Can you work these out from the model? Positions are in its coordinate system, mm. A direction names the side the tool comes from. Round coordinates to 2 decimals unless told otherwise and drop trailing zeros. Write each loop counter-clockwise with the first axis right and the second up, starting at its lowest first coordinate (ties: lowest second). Pieces come first, ordered by that corner, then holes. Notation, with made-up numbers: M 33.25,42 L 78.25,42 A13 cw 78.25,65 Z; hole C 42.5,12.25 d10. An arc over 180 degrees is marked long. Answer in a Markdown table with one row per item. Add a question column.
(1) I'm going to push flat-ended pins straight in: pin 1 (3 mm diameter, centred on y = -11, z = 32, fed in from +X); pin 2 (10 mm diameter, centred on x = 9.5, z = 8, fed in from +Y). Where does each tip first touch, or does it pass through?
(2) Suppose I cut it at C-C, the plane x = 12. Write out the boundary of the cut face in (y, z), then the cut area to 3 significant figures.
(3) If we mould it in two halves opening along Z, with no side actions, what happens to faces 3 (the face through (0, -7, 65)), 4 (the face through (32.5, -2, 32)), 5 (the face through (-2.48, -9, 33))? For each: released by +Z, released by -Z, zero draft, split by the parting line, or undercut.
(4) Suppose I cut it at D-D, the plane x = -16.5. Write out the boundary of the cut face in (y, z).
(5) If I drill on probe 1 along Z at (x, y) = (1, -7.75); probe 2 along Y at (x, z) = (24, 32.5); probe 3 along Y at (x, z) = (-1, 17.5), over which ranges is the centre line in solid material (lowest first)?
(6) For faces 1 (the face through (15.25, -7.44, 27.93)), 2 (the face through (0, -15, 32)), which set-ups out of +Z, -Z, +X, -X, +Y, -Y let a thin tool reach every point of the face, with its end or its side?
(7) Suppose I cut it at B-B, the plane z = 32.5. Write out the boundary of the cut face in (x, y), then the cut area to 3 significant figures.
(8) Suppose I cut it at A-A, the plane y = -8.88. Write out the boundary of the cut face in (x, z), then the cut area to 3 significant figures.
from build123d import *

# Parameters (mm, degrees)
SKIZZE1_W                       = 65
SKIZZE1_H                       = 30
AUFSATZ_LINEAR_AUSTRAGEN1_DEPTH = 65
SKIZZE2_R                       = 95
SCHNITT_LINEAR_AUSTRAGEN1_DEPTH = 65
SKIZZE5_R                       = 4.79
SCHNITT_LINEAR_AUSTRAGEN2_DEPTH = 34.98


with BuildPart() as part:
    # Skizze1 → Aufsatz-Linear austragen1 (new body)
    with BuildSketch(Plane.XY):
        Rectangle(SKIZZE1_W, SKIZZE1_H)
    extrude(amount=AUFSATZ_LINEAR_AUSTRAGEN1_DEPTH)

    # Skizze2 → Schnitt-Linear austragen1 (cut)
    with BuildSketch(Plane.XY.offset(65)):
        with Locations((0, 95)):
            Circle(SKIZZE2_R)
    extrude(amount=-SCHNITT_LINEAR_AUSTRAGEN1_DEPTH, mode=Mode.SUBTRACT)

    # Skizze5 → Schnitt-Linear austragen2 (cut)
    with BuildSketch(Plane(origin=(32.5, 0, 0), x_dir=(0, 0, -1), z_dir=(1, 0, 0))):
        with Locations((-32.5, -8.88)):
            Circle(SKIZZE5_R)
    extrude(amount=-SCHNITT_LINEAR_AUSTRAGEN2_DEPTH, mode=Mode.SUBTRACT)


solid = part.part
Calculated:
| question | item | result |
|---|---|---|
| 1 | pin 1 | x = -2.48 |
| 1 | pin 2 | y = 1.11 |
| 2 | outline | M -15,0 L 0.76,0 L 0.76,65 L -15,65 Z; hole C -8.88,32.5 d9.58 |
| 2 | area | 952 mm² |
| 3 | face 3 | released by +Z |
| 3 | face 4 | zero draft |
| 3 | face 5 | undercut |
| 4 | outline | M -15,0 L 1.44,0 L 1.44,65 L -15,65 Z |
| 5 | probe 1 | 0 to 27.85, 37.15 to 65 |
| 5 | probe 2 | -15 to -13.67, -4.09 to 3.08 |
| 5 | probe 3 | -15 to 0.01 |
| 6 | face 1 | +X |
| 6 | face 2 | +Z, -Z, +X, -X, -Y |
| 7 | outline | M -32.5,-15 L 32.5,-15 L 32.5,-13.67 L -2.48,-13.67 L -2.48,-4.09 L 32.5,-4.09 L 32.5,5.73 A95 cw -32.5,5.73 Z |
| 7 | area | 763 mm² |
| 8 | outline | M -32.5,0 L 32.5,0 L 32.5,27.71 L -2.48,27.71 L -2.48,37.29 L 32.5,37.29 L 32.5,65 L -32.5,65 Z |
| 8 | area | 3,890 mm² |
